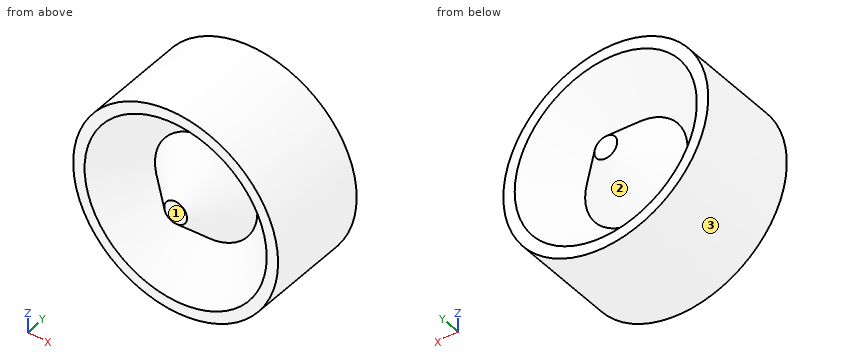
```python
from build123d import *


with BuildPart() as f1:
    # F0 (on Top) → F1 (revolve)
    with BuildSketch(Plane.XY):
        Polygon((4, 0), (0, 0), (0, -36), (4, -36), (18, -22), (32, -36), (36, -36), (36, 0), (32, 0), (18, -14), align=None)
        Polygon((16.343146, -18), (4, -30.343146), (4, -5.656854), align=None, mode=Mode.SUBTRACT)
        Polygon((32, -30.343146), (19.656854, -18), (32, -5.656854), align=None, mode=Mode.SUBTRACT)
        Polygon((4, -5.656854), (4, -30.343146), (16.343146, -18), align=None)
        Polygon((32, -5.656854), (19.656854, -18), (32, -30.343146), align=None)
    revolve(axis=Axis((0, -18, 0), (0, -1, 0)))


solid = f1.part
```
Can you work these out from the model? Positions are in its coordinate system, mm. Face numbers are marked on the shaded views. Give positions to 0.01 mm unless a question says otherwise; leave off trailing zeros. Order: outer loops, then holes, each group sorted by start corner. A loop starts at its lowest first (then second) coordinate and runs counter-clockwise, first axis right, second up. Notation, with made-up numbers: M -29,-31.5 L 9,-31.5 A27 cw 9,-7.5 Z; hole C 53.5,68 d1. An arc over 180 degrees is marked long. Write item = value, one per line. Start each with the question number.
Q1. Suppose I cut it at A-A (y = -27.5). Write out the boundary of the cut face in (x, z).
Q2. Will these pins go through, and if not, where does the flat tip stop? pin 1 Ø4 at (y, z) = (-6, -23.5) entering from +X; pin 2 Ø2 at (x, y) = (-25.5, -22) entering from +Z; pin 3 Ø5 at (x, y) = (-3.5, -32) entering from -Z.
Q3. Suppose I cut it at B-B (x = 0). Write out the boundary of the cut face in (y, z), plus the area to 3 significant figures.
Q4. Suppose I cut it at C-C (z = 0). Write out the boundary of the cut face in (x, y), plus the area to 3 significant figures.
Q5. I need wall thicknesses on probe 1 along X at (y, z) = (-31, -8); probe 2 along Z at (x, y) = (-1, -26); probe 3 along Z at (x, y) = (-12, -11). Which ranges of each line are inside material? Lowest first, please. Write a range as [from, to].
Q6. Suppose I cut it at D-D (y = -3). Write out the boundary of the cut face in (x, z).
Q7. We'd pull the mould along X, two halves only. Please class the marked faces 1, 2 and 3: pulls with the +X half, pulls with the -X half, needs draft (parallel to the pull), parting line crosses it, or undercut.
Check result:
q1.outline = C 0,0 d72; C 0,0 d25; hole C 0,0 d47
q2.pin_1 = 28.87
q2.pin_2 = 26.38
q2.pin_3 = -35.99
q3.outline = M -36,-36 L 0,-36 L 0,-32 L -14,-18 L 0,-4 L 0,4 L -14,18 L 0,32 L 0,36 L -36,36 L -36,32 L -22,18 L -36,4 L -36,-4 L -22,-18 L -36,-32 Z
q3.area = 1,810 mm2
q4.outline = M -36,-36 L -32,-36 L -18,-22 L -4,-36 L 4,-36 L 18,-22 L 32,-36 L 36,-36 L 36,0 L 32,0 L 18,-14 L 4,0 L -4,0 L -18,-14 L -32,0 L -36,0 Z
q4.area = 1,810 mm2
q5.probe_1 = [-35.1, -25.79], [-4.12, 4.12], [25.79, 35.1]
q5.probe_2 = [-35.99, -21.98], [-13.96, 13.96], [21.98, 35.99]
q5.probe_3 = [-33.94, -17.23], [-9, 9], [17.23, 33.94]
q6.outline = C 0,0 d72; C 0,0 d14; hole C 0,0 d58
q7.face_1 = needs draft
q7.face_2 = undercut
q7.face_3 = parting line crosses it
